Part print with two shaded views. Sizes in mm from the minimum x, y, z corner. A direction names the side the tool comes from. Give positions to 0.01 mm unless a question says otherwise; leave off trailing zeros. Write each loop counter-clockwise with the first axis right and the second up, starting at its lowest first coordinate (ties: lowest second). Pieces come first, ordered by that corner, then holes.
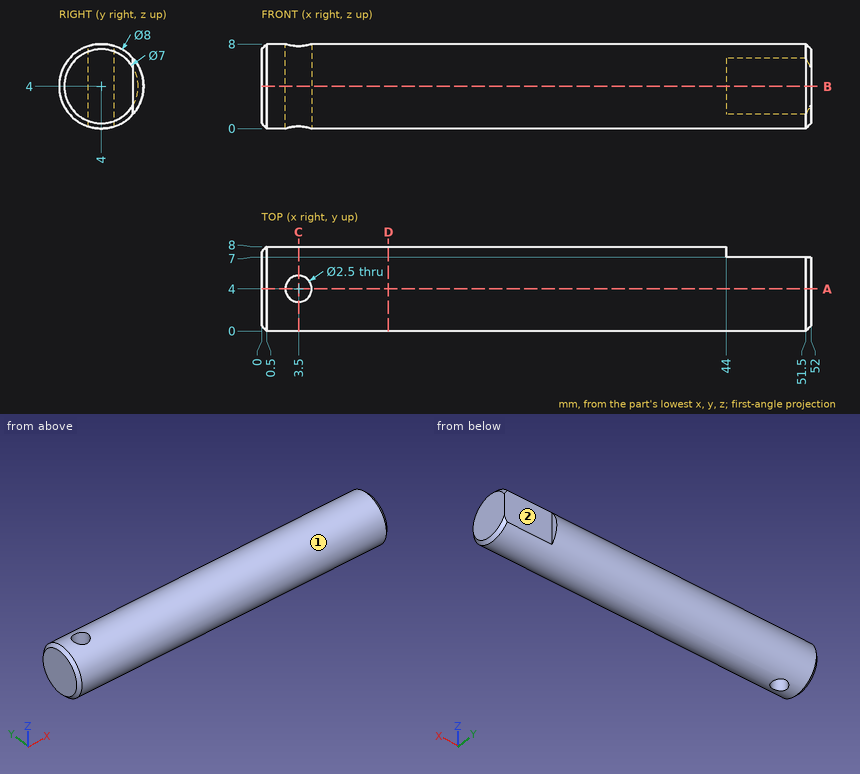
1) 3-axis set-ups, long thin cutter, end or side, ignore diameter. For the marked faces 1 and 2: which of +Z, -Z, +X, -X, +Y, -Y reach the whole face in a straight line?
Answers follow:
face 1: +X, -X
face 2: +Z, -Z, +X, +Y
2) Saw through at C-C, the plane x = 3.5. Write the cut outline in (y, z), then the cut area to 3 significant figures.
Answers follow:
outline: (2.75, 0.2) - (2.75, 7.8) arc R4 ccw to start; (5.25, 0.2) arc R4 ccw to (5.25, 7.8) - close
area: 30.6 mm2
3) Saw through at A-A, the plane y = 4. Write the cut outline in (x, z), then the cut area to 4 significant figures.
Answers follow:
outline: (0, 0.5) - (0.5, 0) - (2.25, 0) - (2.25, 8) - (0.5, 8) - (0, 7.5) - close; (4.75, 0) - (51.5, 0) - (52, 0.5) - (52, 7.5) - (51.5, 8) - (4.75, 8) - close
area: 395.5 mm2
4) Wall check: L1, parallel to Y at x = 3.5, z = 4.25; L2, parallel to X at y = 4.75, z = 5; L3, parallel to Y at x = 3.5, z = 5.5. Give the ranges that are in metal, low to high.
Answers follow:
L1: y = 0.01 to 2.75, 5.25 to 7.99
L2: x = 0 to 2.5, 4.5 to 52
L3: y = 0.29 to 2.75, 5.25 to 7.71
5) Saw through at D-D, the plane x = 12. Write the cut outline in (y, z), then the cut area to 3 significant figures.
Answers follow:
outline: circle Ø8 at (4, 4)
area: 50.3 mm2
6) Saw through at B-B, the plane z = 4. Write the cut outline in (x, y), then the cut area to 3 significant figures.
Answers follow:
outline: (0, 0.5) - (0.5, 0) - (51.5, 0) - (52, 0.5) - (52, 7) - (44, 7) - (44, 8) - (0.5, 8) - (0, 7.5) - close; hole circle Ø2.5 at (3.5, 4)
area: 403 mm2
7) Pin check, flat tips, straight feed: pin 1 Ø4 at (x, z) = (47, 3) entering from +Y; pin 2 Ø2 at (x, z) = (18, 5.5) entering from -Y; pin 3 Ø2 at (x, z) = (16, 2) entering from -Y. Stop position of each tip, or through.
Answers follow:
pin 1: stops at y = 7
pin 2: stops at y = 0.03
pin 3: stops at y = 0.13
